The figure shows three views and two pictorial views of one solid part (mm, origin at its lowest corner). Answer the questions. Coordinates: 2 decimals unless noted, no trailing zeros. Loops run counter-clockwise (first coordinate to the right, second up) from the corner with the lowest first, then second, coordinate; pieces in that order, holes last. Notation, with made-up numbers: (82, 40.25) - (109, 40.25) arc R10 ccw to (109, 59.25) - close; hole circle Ø2 at (26.25, 2.25). An arc over 180 degrees is marked (long way). Return JSON: item names as keys, results as strings. Group by question number.
1. Section A-A (x = 14.25) is taken. Write down the section's boundary in (y, z).
2. Section C-C (y = 42) is taken. Write down the section's boundary in (x, z).
3. Each of these flat-tipped pins is pushed along its axis until it touches: P1, Ø5.5, axis at y = 66, z = 9, coming from the +X side; P2, Ø4, axis at y = 64, z = 10, coming from the -X side; P3, Ø2.5, axis at y = 19.5, z = 45.5, coming from the +X side. Where does it stop, or does it pass through?
4. Section B-B (z = 50) is taken. Write down the section's boundary in (x, y).
5. Find the intervals of material crossed by line 1 along Z through (x, y) = (11.6, 20); line 2 along Z through (x, y) = (12.25, 64); line 3 along X through (y, z) = (44, 43.5), in increasing order.
6. Section D-D (z = 14.5) is taken. Write down the section's boundary in (x, y).
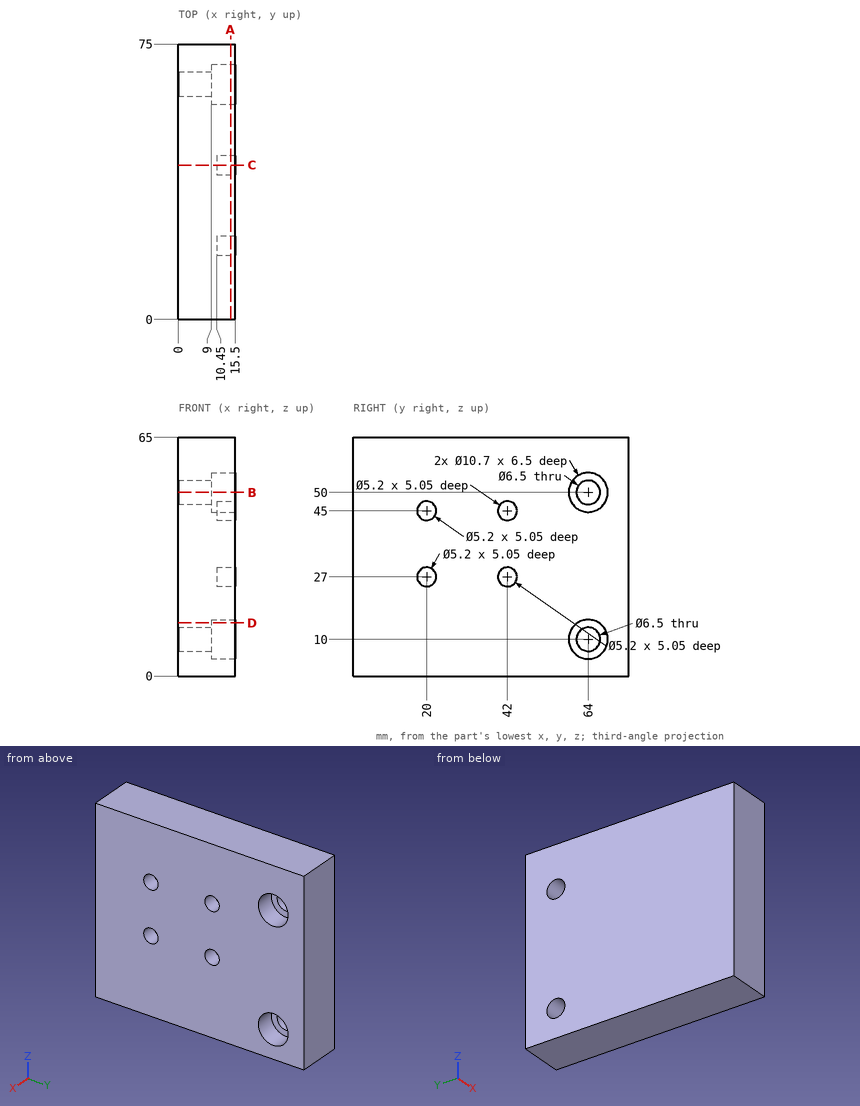
The answers:
{
 "1": {"outline": "(0, 0) - (75, 0) - (75, 65) - (0, 65) - close; hole circle Ø5.2 at (20, 27); hole circle Ø5.2 at (20, 45); hole circle Ø5.2 at (42, 27); hole circle Ø5.2 at (42, 45); hole circle Ø10.7 at (64, 10); hole circle Ø10.7 at (64, 50)"},
 "2": {"outline": "(0, 0) - (15.5, 0) - (15.5, 24.4) - (10.45, 24.4) - (10.45, 29.6) - (15.5, 29.6) - (15.5, 42.4) - (10.45, 42.4) - (10.45, 47.6) - (15.5, 47.6) - (15.5, 65) - (0, 65) - close"},
 "3": {"P1": "stops at x = 9", "P2": "passes through", "P3": "stops at x = 10.45"},
 "4": {"outline": "(0, 0) - (15.5, 0) - (15.5, 58.65) - (9, 58.65) - (9, 60.75) - (0, 60.75) - close; (0, 67.25) - (9, 67.25) - (9, 69.35) - (15.5, 69.35) - (15.5, 75) - (0, 75) - close"},
 "5": {"line 1": "z = 0 to 24.4, 29.6 to 42.4, 47.6 to 65", "line 2": "z = 0 to 4.65, 15.35 to 44.65, 55.35 to 65", "line 3": "x = 0 to 10.45"},
 "6": {"outline": "(0, 0) - (15.5, 0) - (15.5, 61.11) - (9, 61.11) - (9, 66.89) - (15.5, 66.89) - (15.5, 75) - (0, 75) - close"}
}
